Geometry check sheet. Reference: the model listing, model coordinates, mm. A direction names the side the tool comes from. Give positions to 0.01 mm unless a question says otherwise; leave off trailing zeros. Write each loop counter-clockwise with the first axis right and the second up, starting at its lowest first coordinate (ties: lowest second). Pieces come first, ordered by that corner, then holes. Notation, with made-up numbers: (48, 12) -> (90, 12) arc R17 cw to (90, 30) -> close; hole circle Ø10 at (-19.5, 64.5). An arc over 180 degrees is marked (long way). Write item = value, one per line. Start each with the question number.
1. Depth check by flat-ended pin: P1, Ø6.5, axis at x = -74.5, y = -14, coming from the -Z side; P2, Ø2, axis at x = -524.5, z = 228, coming from the -Y side; P3, Ø6.5, axis at y = -10, z = 88.5, coming from the +X side. Enter the tip coordinate at first touch or a pass-through.
2. Mould release check, pull along X, two halves, no side actions. Record for faces 6 (the flat face through (-6.35, -12, 112)), 7 (the flat face through (-314.6, -18.034, 18.7)), 8 (the flat face through (-121.867, -11.773, 213.449)): pulls with the +X half, pulls with the -X half, needs draft (parallel to the pull), parting line crosses it, or undercut.
3. Set-up check for faces 1 (the flat face through (-85, -12, 214.557)), 2 (the cylindrical face through (-26.69, -11.77, 26.29)), 3 (the flat face through (-351, -12, 219.71)), 4 (the flat face through (-296, -12, 6.35)), 5 (the flat face through (-577.85, -12, 112)): record each of +Z, -Z, +X, -X, +Y, -Y from which the full face is reachable in a straight line by a thin tool's end or side.
4. Thickness scan on line 1 along Z through (x, y) = (-330, -16); line 2 along X through (y, z) = (-12.75, 75.5); line 3 along Y through (x, z) = (-316, 27). Record the ranges inside material, lowest first.
5. Cross-section at A-A, the plane y = -13.5. Record the cut outline in (x, z), plus the area to 3 significant figures.
```python
from build123d import *

# Parameters (mm, degrees)
F0_W     = 584.2
F0_H     = 219.71
F1_DEPTH = 5.334
F2_W     = 571.5
F2_H     = 213.36
F2_W_2   = 546.1
F2_H_2   = 187.96
F3_DEPTH = 12.7
F4_R     = 25.4
F6_DEPTH = 12.7
F8_DEPTH = 5.334
F9_DEPTH = 5.334


# Not quite as in the source:
# - a feature names something its author has since deleted; it is built from what else it names


with BuildPart() as f1:
    # F0 (on Front) → F1 (new body)
    with BuildSketch(Plane.XZ):
        with Locations((-292.1, 109.855)):
            Rectangle(F0_W, F0_H)
    extrude(amount=F1_DEPTH)

    # F2 (on face) → F3 (join)
    with BuildSketch(Plane.XZ.offset(5.334)):
        with Locations((-292.1, 113.03)):
            Rectangle(F2_W, F2_H)
        with Locations((-292.1, 113.03)):
            Rectangle(F2_W_2, F2_H_2, mode=Mode.SUBTRACT)
    extrude(amount=F3_DEPTH)

    # F4
    f4_edges = [f1.edges().sort_by_distance(p)[0] for p in [
        (-565.15, -11.684, 207.01),
        (-19.05, -11.684, 207.01),
        (-19.05, -11.684, 19.05),
        (-565.15, -11.684, 19.05),
    ]]
    fillet(f4_edges, radius=F4_R)

    # F5 (on face) → F6 (cut)
    with BuildSketch(Plane.XZ.offset(18.034)):
        Polygon((-118.11, 219.71), (-125.73, 207.01), (-118.11, 207.01), (-113.5820166854, 214.5566388576), (-110.49, 219.71), align=None)
        Polygon((-56.5979833146, 214.5566388576), (-52.07, 207.01), (-44.45, 207.01), (-52.07, 219.71), (-59.69, 219.71), align=None)
        Polygon((-59.69, 219.71), (-110.49, 219.71), (-113.5820166854, 214.5566388576), (-56.5979833146, 214.5566388576), align=None)
    extrude(amount=-F6_DEPTH, mode=Mode.SUBTRACT)

    # F7 (on face) → F8 (cut)
    with BuildSketch(Plane(origin=(0, 0, 0), x_dir=(-1, 0, 0), z_dir=(0, 1, 0))):
        with BuildLine():
            add(Edge.make_bspline(
                [(292.1, 6.35), (289.8878914708, 4.2388101088), (287.6757829415, 2.1276202176), (285.3383261504, 0)],
                knots=[0, 0, 0, 0, 0.0566650496, 0.0566650496, 0.0566650496, 0.0566650496], degree=3))
            Line((285.3383261504, 0), (292.1, 0))
            Line((292.1, 0), (292.1, 6.35))
        make_face()
        with BuildLine():
            add(Edge.make_bspline(
                [(292.1, 6.35), (294.3115112442, 4.2388053382), (296.5230224884, 2.1276106765), (298.8599853109, 0)],
                knots=[0, 0, 0, 0, 0.056662645, 0.056662645, 0.056662645, 0.056662645], degree=3))
            Line((292.1, 6.35), (292.1, 0))
            Line((292.1, 0), (298.8599853109, 0))
        make_face()
    extrude(amount=-F8_DEPTH, mode=Mode.SUBTRACT)

    # F7 (on face) → F9 (join)
    with BuildSketch(Plane(origin=(0, 0, 0), x_dir=(-1, 0, 0), z_dir=(0, 1, 0))):
        with BuildLine():
            Line((285.3383261504, 0), (0, 0))
            add(Edge.make_bspline(
                [(35.5548654074, -18.4164866805), (23.6750755263, -12.5314961521), (11.8375377632, -6.265748076), (0, 0)],
                knots=[0.8952858021, 0.8952858021, 0.8952858021, 0.8952858021, 1, 1, 1, 1], degree=3))
            Line((35.5548654074, -18.4164866805), (260.35, -18.4164866805))
            add(Edge.make_bspline(
                [(285.3383261504, 0), (278.8607301271, -5.8960937002), (271.4205053001, -11.9183662972), (260.35, -18.4164866805)],
                knots=[0.0566650496, 0.0566650496, 0.0566650496, 0.0566650496, 0.2136961022, 0.2136961022, 0.2136961022, 0.2136961022], degree=3))
        make_face()
        with BuildLine():
            add(Edge.make_bspline(
                [(0, 0), (-2.7059325948, 17.274832353), (-4.5181928473, 42.574440276), (-5.08, 63.5)],
                knots=[0, 0, 0, 0, 0.5267133936, 0.5267133936, 0.5267133936, 0.5267133936], degree=3))
            Line((0, 0), (0, 219.71))
            add(Edge.make_bspline(
                [(0, 219.71), (-2.907575848, 216.0546733014), (-4.393729889, 212.1257933571), (-5.08, 208.0429754021)],
                knots=[0.6401685719, 0.6401685719, 0.6401685719, 0.6401685719, 0.7975102285, 0.7975102285, 0.7975102285, 0.7975102285], degree=3))
            Line((-5.08, 208.0429754021), (-5.08, 191.77))
            Line((-5.08, 191.77), (-5.08, 114.935))
            Line((-5.08, 114.935), (-5.08, 63.5))
        make_face()
        with BuildLine():
            Line((260.35, -18.4164866805), (35.5548654074, -18.4164866805))
            add(Edge.make_bspline(
                [(143.5928555626, -50.8), (106.470496214, -50.0055886792), (70.8264502644, -35.8892656507), (35.5548654074, -18.4164866805)],
                knots=[0.5843850409, 0.5843850409, 0.5843850409, 0.5843850409, 0.8952858021, 0.8952858021, 0.8952858021, 0.8952858021], degree=3))
            Line((143.5928555626, -50.8), (150.3785817486, -50.8))
            add(Edge.make_bspline(
                [(260.35, -18.4164866805), (235.5497171967, -32.973656279), (192.5306851802, -49.9188924594), (150.3785817486, -50.8)],
                knots=[0.2136961022, 0.2136961022, 0.2136961022, 0.2136961022, 0.5654790071, 0.5654790071, 0.5654790071, 0.5654790071], degree=3))
        make_face()
        with BuildLine():
            add(Edge.make_bspline(
                [(11.5967126237, 229.2998559787), (6.6790583406, 226.3057112292), (2.7183257178, 223.1274064895), (0, 219.71)],
                knots=[0.4930680682, 0.4930680682, 0.4930680682, 0.4930680682, 0.6401685719, 0.6401685719, 0.6401685719, 0.6401685719], degree=3))
            Line((0, 219.71), (292.1, 219.71))
            Line((292.1, 219.71), (11.5967126237, 229.2998559787))
        make_face()
        with BuildLine():
            add(Edge.make_bspline(
                [(12.5483744012, 229.87), (12.2273175537, 229.6806902818), (11.9100723395, 229.4906470132), (11.5967126237, 229.2998559787)],
                knots=[0.4836946212, 0.4836946212, 0.4836946212, 0.4836946212, 0.4930680682, 0.4930680682, 0.4930680682, 0.4930680682], degree=3))
            Line((11.5967126237, 229.2998559787), (292.1, 219.71))
            Line((292.1, 219.71), (573.5876283802, 229.3335086626))
            add(Edge.make_bspline(
                [(572.7896932404, 229.87), (573.0585490403, 229.6916783135), (573.3245454934, 229.5128510633), (573.5876283802, 229.3335086626)],
                knots=[0.4655830842, 0.4655830842, 0.4655830842, 0.4655830842, 0.4744116019, 0.4744116019, 0.4744116019, 0.4744116019], degree=3))
            Line((572.7896932404, 229.87), (514.35, 229.87))
            Line((514.35, 229.87), (292.1, 229.87))
            Line((292.1, 229.87), (82.55, 229.87))
            Line((82.55, 229.87), (12.5483744012, 229.87))
        make_face()
        with BuildLine():
            Line((573.5876283802, 229.3335086626), (292.1, 219.71))
            Line((292.1, 219.71), (584.2, 219.71))
            add(Edge.make_bspline(
                [(573.5876283802, 229.3335086626), (578.0527057549, 226.2896858373), (581.6785208511, 223.0974722581), (584.2, 219.71)],
                knots=[0.4744116019, 0.4744116019, 0.4744116019, 0.4744116019, 0.6242503674, 0.6242503674, 0.6242503674, 0.6242503674], degree=3))
        make_face()
        with BuildLine():
            add(Edge.make_bspline(
                [(298.8599853109, 0), (305.3364495341, -5.8962831133), (312.7764065366, -11.9186444461), (323.85, -18.4164866805)],
                knots=[0.056662645, 0.056662645, 0.056662645, 0.056662645, 0.2136927825, 0.2136927825, 0.2136927825, 0.2136927825], degree=3))
            Line((323.85, -18.4164866805), (548.6673215949, -18.4164866805))
            add(Edge.make_bspline(
                [(548.6673215949, -18.4164866805), (560.540064076, -12.5314899408), (572.370032038, -6.2657449704), (584.2, 0)],
                knots=[0.8952964295, 0.8952964295, 0.8952964295, 0.8952964295, 1, 1, 1, 1], degree=3))
            Line((584.2, 0), (298.8599853109, 0))
        make_face()
        with BuildLine():
            Line((548.6673215949, -18.4164866805), (323.85, -18.4164866805))
            add(Edge.make_bspline(
                [(323.85, -18.4164866805), (348.6543054028, -32.9713340996), (391.6899454814, -49.9118498543), (433.8458201185, -50.8)],
                knots=[0.2136927825, 0.2136927825, 0.2136927825, 0.2136927825, 0.5654325768, 0.5654325768, 0.5654325768, 0.5654325768], degree=3))
            Line((433.8458201185, -50.8), (440.69, -50.8))
            add(Edge.make_bspline(
                [(440.69, -50.8), (477.8051745876, -49.9992725657), (513.4246952416, -35.8853016167), (548.6673215949, -18.4164866805)],
                knots=[0.5844980763, 0.5844980763, 0.5844980763, 0.5844980763, 0.8952964295, 0.8952964295, 0.8952964295, 0.8952964295], degree=3))
        make_face()
        with BuildLine():
            add(Edge.make_bspline(
                [(82.55, 255.27), (55.8328777889, 247.4544406939), (29.1157555777, 239.6388813877), (12.5483744012, 229.87)],
                knots=[0, 0, 0, 0, 0.4836946212, 0.4836946212, 0.4836946212, 0.4836946212], degree=3))
            Line((12.5483744012, 229.87), (82.55, 229.87))
            Line((82.55, 229.87), (82.55, 255.27))
        make_face()
        with BuildLine():
            add(Edge.make_bspline(
                [(584.2, 219.71), (587.2466521414, 215.6169859397), (588.681040168, 211.2389059428), (589.28, 206.7131131)],
                knots=[0.6242503674, 0.6242503674, 0.6242503674, 0.6242503674, 0.8052975103, 0.8052975103, 0.8052975103, 0.8052975103], degree=3))
            Line((584.2, 219.71), (584.2, 0))
            add(Edge.make_bspline(
                [(584.2, 0), (587.0231389999, 19.4493960589), (588.7459289581, 43.301401327), (589.28, 63.5)],
                knots=[0, 0, 0, 0, 0.5267133936, 0.5267133936, 0.5267133936, 0.5267133936], degree=3))
            Line((589.28, 63.5), (589.28, 114.935))
            Line((589.28, 114.935), (589.28, 191.77))
            Line((589.28, 191.77), (589.28, 206.7131131))
        make_face()
        with BuildLine():
            Line((82.55, 255.27), (82.55, 229.87))
            Line((82.55, 229.87), (292.1, 229.87))
            Line((292.1, 229.87), (292.1, 306.07))
            add(Edge.make_bspline(
                [(292.1, 306.07), (222.25, 289.1366666667), (152.4, 272.2033333333), (82.55, 255.27)],
                knots=[0, 0, 0, 0, 215.6196709486, 215.6196709486, 215.6196709486, 215.6196709486], degree=3))
        make_face()
        with BuildLine():
            Line((514.35, 229.87), (572.7896932404, 229.87))
            add(Edge.make_bspline(
                [(514.35, 255.27), (536.4806207919, 247.2720101715), (558.6112415838, 239.274020343), (572.7896932404, 229.87)],
                knots=[0, 0, 0, 0, 0.4655830842, 0.4655830842, 0.4655830842, 0.4655830842], degree=3))
            Line((514.35, 255.27), (514.35, 229.87))
        make_face()
        with BuildLine():
            Line((292.1, 306.07), (292.1, 229.87))
            Line((292.1, 229.87), (514.35, 229.87))
            Line((514.35, 229.87), (514.35, 255.27))
            add(Edge.make_bspline(
                [(514.35, 255.27), (440.2666666667, 272.2033333333), (366.1833333333, 289.1366666667), (292.1, 306.07)],
                knots=[0, 0, 0, 0, 227.9818030019, 227.9818030019, 227.9818030019, 227.9818030019], degree=3))
        make_face()
    extrude(amount=-F9_DEPTH)


solid = f1.part
```
Answers:
q1.P1 = 6.35
q1.P2 = -5.33
q1.P3 = -6.35
q2.face_6 = pulls with the +X half
q2.face_7 = needs draft
q2.face_8 = undercut
q3.face_1 = +Z, -Y
q3.face_2 = -Y
q3.face_3 = +Z, +X, -X, -Y
q3.face_4 = -Z, +X, -X, -Y
q3.face_5 = +Z, -Z, -X, -Y
q4.line_1 = 6.35 to 19.05, 207.01 to 219.71
q4.line_2 = -577.85 to -565.15, -19.05 to -6.35
q4.line_3 = -5.33 to 0
q5.outline = (-577.85, 6.35) -> (-6.35, 6.35) -> (-6.35, 219.71) -> (-52.07, 219.71) -> (-44.45, 207.01) arc R25.4 cw to (-19.05, 181.61) -> (-19.05, 44.45) arc R25.4 cw to (-44.45, 19.05) -> (-539.75, 19.05) arc R25.4 cw to (-565.15, 44.45) -> (-565.15, 181.61) arc R25.4 cw to (-539.75, 207.01) -> (-125.73, 207.01) -> (-118.11, 219.71) -> (-577.85, 219.71) -> close; (-118.11, 207.01) -> (-52.07, 207.01) -> (-56.6, 214.56) -> (-113.58, 214.56) -> close
q5.area = 19,400 mm^2
